Input: part model. Units: mm. Frame: model coordinates. Face numbers are marked on the shaded views. A direction names the side the tool comes from. Coordinates: 2 decimals unless noted, no trailing zeros. Loops run counter-clockwise (first coordinate to the right, second up) from the corner with the lowest first, then second, coordinate; pieces in that order, holes last. Notation, with made-up numbers: (26.5, -33) - (69.5, -33) arc R17 cw to (69.5, -3) - close; hole circle Ø5 at (80.5, 73.5). An arc over 180 degrees is marked (long way). Use a Markdown table: item, result. Add a question column.
1. Section query B-B on x = -72. Return the cut outline in (y, z), then the cut area to 3 significant figures.
2. Section query D-D on x = 76. Return the cut outline in (y, z).
3. Section query C-C on y = 74.5. State how many separate pieces and enclosed holes the cut face has, then the cut area to 3 significant figures.
4. Access query for the marked faces 1 and 2. Directions: +Z, -Z, +X, -X, +Y, -Y. A direction counts if a zero-diameter tool reaches every point of the face in a straight line with its end or side. Return the directions, or none.
5. Contact query for flat-ended pins moving along their axis: P1, Ø7.5, axis at x = -84.5, y = 37.5, coming from the -Z side; P2, Ø2, axis at y = 67, z = 16.5, coming from the -X side; P3, Ø21.5, axis at x = 82.6, z = 60.4, coming from the +Y side; P4, Ø5, axis at y = 93.5, z = 24.5, coming from the +X side. Output: stop coordinate, or through.
6. Section query A-A on z = 60.4. Return the cut outline in (x, y), then the cut area to 3 significant figures.
7. Ray query, L1, parallel to X at y = 58, z = 60.4; L2, parallel to X at y = 16, z = 21; L3, parallel to Z at x = 26.5, y = 35.5. Return the intervals inside material, ascending. Write a range as [from, to].
8. Draft query along Z for the marked faces 3, 4, 5 and 6. Return one class per face: released by +Z, released by -Z, zero draft, split by the parting line, or undercut.
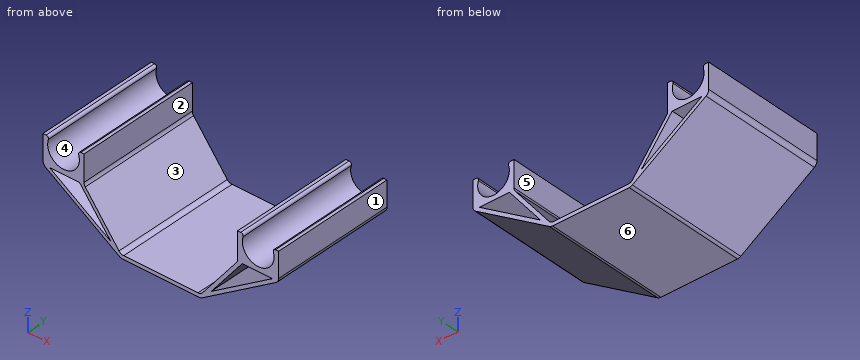
```python
from build123d import *

# Parameters (mm, degrees)
BOSS_EXTRUDE1_DEPTH = 105.5
FILLET1_R           = 5


with BuildPart() as part:
    # Sketch1 → Boss-Extrude1 (new body)
    with BuildSketch(Plane(origin=(0, 0, 0), x_dir=(1, 0, 0), z_dir=(0, 1, 0))):
        with BuildLine():
            Line((0, 0), (-34, 0))
            Line((-34, 0), (-100, -43))
            Line((-100, -43), (-100, -66.97))
            Line((-100, -66.97), (-97.358644924, -66.97))
            ThreePointArc((-97.358644924, -66.97), (-95.748804634, -66.156766295), (-95.448140727, -64.378414239))
            ThreePointArc((-95.448140727, -64.378414239), (-82.6, -46.95), (-69.751859273, -64.378414239))
            ThreePointArc((-69.751859273, -64.378414239), (-69.451195366, -66.156766295), (-67.841355076, -66.97))
            Line((-67.841355076, -66.97), (-65.2, -66.97))
            Line((-65.2, -66.97), (-65.2, -43))
            Line((-65.2, -43), (-34, -3))
            Line((-34, -3), (0, -3))
            Line((0, -3), (0, 0))
        make_face()
        Polygon((-69.004681327, -43), (-94.504291462, -43), (-42.656655328, -9.220479488), align=None, mode=Mode.SUBTRACT)
    boss_extrude1 = extrude(amount=BOSS_EXTRUDE1_DEPTH)

    # Mirror1: Boss-Extrude1 across plane
    add(boss_extrude1.mirror(Plane(origin=(0, 105.5, 3), x_dir=(0, 0, 1), z_dir=(-1, 0, 0))))

    # Fillet1
    fillet1_edges = [part.edges().sort_by_distance(p)[0] for p in [
        (-34, 52.75, 3),
        (-65.2, 52.75, 43),
        (-100, 52.75, 43),
        (-34, 52.75, 0),
        (34, 52.75, 3),
        (65.2, 52.75, 43),
        (100, 52.75, 43),
        (34, 52.75, 0),
    ]]
    fillet(fillet1_edges, radius=FILLET1_R)


solid = part.part
```
Resolved:
| question | item | result |
|---|---|---|
| 1 | outline | (0, 24.76) - (105.5, 24.76) - (105.5, 28.34) - (0, 28.34) - close; (0, 43) - (105.5, 43) - (105.5, 52.12) - (0, 52.12) - close |
| 1 | area | 1,340 mm² |
| 2 | outline | (0, 27.36) - (105.5, 27.36) - (105.5, 30.94) - (0, 30.94) - close; (0, 43) - (105.5, 43) - (105.5, 48.68) - (0, 48.68) - close |
| 3 | separate pieces | 1 |
| 3 | enclosed holes | 2 |
| 3 | area | 1,690 mm² |
| 4 | face 1 | +Z, -Z, +X, +Y, -Y |
| 4 | face 2 | +Z, +Y, -Y |
| 5 | P1 | z = 30.46 |
| 5 | P2 | x = -60.86 |
| 5 | P3 | through |
| 5 | P4 | x = 75.44 |
| 6 | outline | (-100, 0) - (-96.05, 0) - (-96.05, 105.5) - (-100, 105.5) - close; (-69.15, 0) - (-65.2, 0) - (-65.2, 105.5) - (-69.15, 105.5) - close; (65.2, 0) - (69.15, 0) - (69.15, 105.5) - (65.2, 105.5) - close; (96.05, 0) - (100, 0) - (100, 105.5) - (96.05, 105.5) - close |
| 6 | area | 1,670 mm² |
| 7 | L1 | [-100, -96.05], [-69.15, -65.2], [65.2, 69.15], [96.05, 100] |
| 7 | L2 | [-66.23, -60.74], [-51.84, -48.04], [48.04, 51.84], [60.74, 66.23] |
| 7 | L3 | [0, 3] |
| 8 | face 3 | released by +Z |
| 8 | face 4 | undercut |
| 8 | face 5 | zero draft |
| 8 | face 6 | released by -Z |
